The listing builds one solid part. Answer for the finished solid, in the listing's coordinates (mm). A direction names the side the tool comes from. Round coordinates to 2 decimals unless told otherwise and drop trailing zeros. Loops run counter-clockwise (first coordinate to the right, second up) from the corner with the lowest first, then second, coordinate; pieces in that order, holes last. Notation, with made-up numbers: (21.5, 4.25) -> (36.5, 4.25) arc R9 ccw to (36.5, 14.25) -> close; hole circle Ø5 at (52, -5.5). An arc over 180 degrees is marked (long way). Use a Markdown table: item, result. Add a question column.
Q1. Section A-A on z = 39 is taken. Give the vertices of the cut face in (x, y), then the cut area to 3 significant figures.
Q2. Which of the six approach directions +Z, -Z, +X, -X, +Y, -Y give full straight-line access (tool end or side, diameter ignored) to faces 5 (the flat face through (0, 0.4, 84)), 6 (the flat face through (0, 0.4, 0)), 7 (the flat face through (0, 0, 41)), 8 (the flat face through (-8, 0, 41)), 9 (the flat face through (8, 0, 41))?
Q3. Given pin 1 Ø1.5 at (y, z) = (-3, 22.5) entering from -X; pin 2 Ø0.7 at (x, z) = (-8, 31) entering from -Y; pin 3 Ø0.6 at (y, z) = (-0.5, 57) entering from +X, each flat-ended and moving along its own axis, determine where each tip first touches the part or whether it passes through.
Q4. For a pull along X with two mould halves and no side action, classify faces 1 (the flat face through (7.203, -2.909, 41.412)), 2 (the flat face through (-6, -2, 41)), 3 (the flat face through (-7.196, -2.936, 41.412)), 4 (the flat face through (0, 1, 41)) as released by +X, released by -X, zero draft, split by the parting line, or undercut.
Q5. Consider line 1 (X direction, y = -0.2, z = 32); line 2 (Y direction, x = 3, z = 10.5); line 3 (X direction, y = -2.9, z = 66.5). Determine where each line is inside the solid, lowest interval first.
Q6. Section B-B on x = -1.25 is taken. Give the vertices of the cut face in (y, z), then the cut area to 3 significant figures.
from build123d import *

# Parameters (mm, degrees)
BOSS_EXTRUDE1_DEPTH = 84
FILLET1_R           = 0.3


with BuildPart() as part:
    # Sketch1 → Boss-Extrude1 (new body)
    with BuildSketch(Plane.XY):
        Polygon((-8.3, 1), (8.3, 1), (8.3, 0), (7, 0), (7, -1.3), (7.5, -1.8), (6.883716857, -4.1), (6, -4.1), (6, 0), (-6, 0), (-6, -4.1), (-6.883716857, -4.1), (-7.5, -1.8), (-7, -1.3), (-7, 0), (-8.3, 0), align=None)
    extrude(amount=BOSS_EXTRUDE1_DEPTH)

    # Fillet1
    fillet1_edges = [part.edges().sort_by_distance(p)[0] for p in [
        (-8.3, 1, 42),
        (8.3, 1, 42),
        (7, -1.3, 42),
        (7.5, -1.8, 42),
        (6.883716857, -4.1, 42),
        (6, -4.1, 42),
        (6, 0, 42),
        (-6, 0, 42),
        (-6, -4.1, 42),
        (-6.883716857, -4.1, 42),
        (-7.5, -1.8, 42),
        (-7, -1.3, 42),
    ]]
    fillet(fillet1_edges, radius=FILLET1_R)


solid = part.part
Checked values:
| question | item | result |
|---|---|---|
| 1 | outline | (-8.3, 0) -> (-7, 0) -> (-7, -1.18) arc R0.3 cw to (-7.09, -1.39) -> (-7.38, -1.68) arc R0.3 ccw to (-7.46, -1.97) -> (-6.94, -3.88) arc R0.3 ccw to (-6.65, -4.1) -> (-6.3, -4.1) arc R0.3 ccw to (-6, -3.8) -> (-6, -0.3) arc R0.3 cw to (-5.7, 0) -> (5.7, 0) arc R0.3 cw to (6, -0.3) -> (6, -3.8) arc R0.3 ccw to (6.3, -4.1) -> (6.65, -4.1) arc R0.3 ccw to (6.94, -3.88) -> (7.46, -1.97) arc R0.3 ccw to (7.38, -1.68) -> (7.09, -1.39) arc R0.3 cw to (7, -1.18) -> (7, 0) -> (8.3, 0) -> (8.3, 0.7) arc R0.3 ccw to (8, 1) -> (-8, 1) arc R0.3 ccw to (-8.3, 0.7) -> close |
| 1 | area | 25.9 mm2 |
| 2 | face 5 | +Z, +X, -X, +Y, -Y |
| 2 | face 6 | -Z, +X, -X, +Y, -Y |
| 2 | face 7 | +Z, -Z, -Y |
| 2 | face 8 | +Z, -Z, -X |
| 2 | face 9 | +Z, -Z, +X |
| 3 | pin 1 | stops at x = -7.38 |
| 3 | pin 2 | stops at y = 0 |
| 3 | pin 3 | stops at x = 7 |
| 4 | face 1 | released by +X |
| 4 | face 2 | undercut |
| 4 | face 3 | released by -X |
| 4 | face 4 | zero draft |
| 5 | line 1 | x = -7 to -5.98, 5.98 to 7 |
| 5 | line 2 | y = 0 to 1 |
| 5 | line 3 | x = -7.21 to -6, 6 to 7.21 |
| 6 | outline | (0, 0) -> (1, 0) -> (1, 84) -> (0, 84) -> close |
| 6 | area | 84.0 mm2 |
